```python
from build123d import *

# Parameters (mm, degrees)
BOSS_EXTRUDE1_DEPTH = 50
CUT_EXTRUDE1_REACH  = 64.546
SKETCH2_R           = 2.5
CUT_EXTRUDE2_REACH  = 63.384
SKETCH3_R           = 3
FILLET1_R           = 6


with BuildPart() as part:
    # Sketch1 → Boss-Extrude1 (new, symmetric)
    with BuildSketch(Plane.XY):
        Polygon((0, 34), (0, 0), (22, 0), (22, 6), (6, 6), (6, 34), align=None)
    extrude(amount=BOSS_EXTRUDE1_DEPTH, both=True)

    # Sketch2 → Cut-Extrude1 (cut, up to next)
    with BuildSketch(Plane(origin=(6, 0, 0), x_dir=(0, 0, -1), z_dir=(1, 0, 0)), mode=Mode.PRIVATE) as cut_extrude1_sk1:
        with Locations(Location((-37.5, 22, 0), (0, 0, 90))):
            Circle(SKETCH2_R)
    cut_extrude1_tool1 = extrude(cut_extrude1_sk1.sketch, amount=-CUT_EXTRUDE1_REACH, mode=Mode.PRIVATE) & part.part
    # Sketch2 → Cut-Extrude1 (cut, up to next)
    with BuildSketch(Plane(origin=(6, 0, 0), x_dir=(0, 0, -1), z_dir=(1, 0, 0)), mode=Mode.PRIVATE) as cut_extrude1_sk2:
        with Locations((37.5, 22)):
            Circle(SKETCH2_R)
    cut_extrude1_tool2 = extrude(cut_extrude1_sk2.sketch, amount=-CUT_EXTRUDE1_REACH, mode=Mode.PRIVATE) & part.part
    add(cut_extrude1_tool1.solids().sort_by_distance((6, 22, 37.5))[0], mode=Mode.SUBTRACT)
    add(cut_extrude1_tool2.solids().sort_by_distance((6, 22, -37.5))[0], mode=Mode.SUBTRACT)

    # Sketch3 → Cut-Extrude2 (cut, up to next)
    with BuildSketch(Plane(origin=(0, 6, 0), x_dir=(1, 0, 0), z_dir=(0, 1, 0)), mode=Mode.PRIVATE) as cut_extrude2_sk1:
        with Locations(Location((13.3, 0, 0), (0, 0, 180))):
            Circle(SKETCH3_R)
    cut_extrude2_tool1 = extrude(cut_extrude2_sk1.sketch, amount=-CUT_EXTRUDE2_REACH, mode=Mode.PRIVATE) & part.part
    add(cut_extrude2_tool1.solids().sort_by_distance((13.3, 6, 0))[0], mode=Mode.SUBTRACT)

    # Fillet1
    fillet1_edges = [part.edges().sort_by_distance(p)[0] for p in [
        (22, 3, 50),
        (3, 34, 50),
        (22, 3, -50),
        (3, 34, -50),
    ]]
    fillet(fillet1_edges, radius=FILLET1_R)


solid = part.part
```
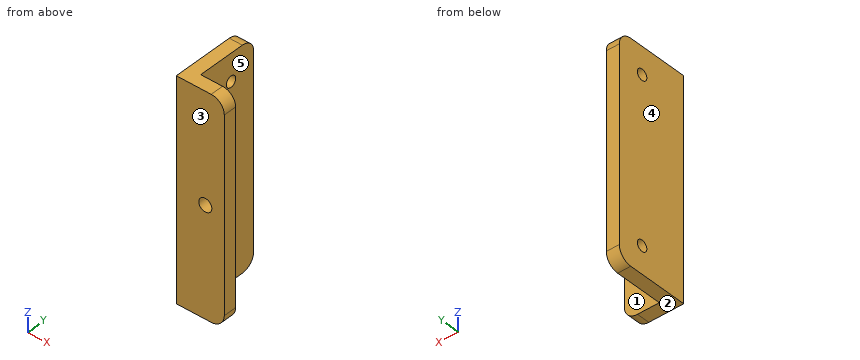
Input: part model. Units: mm. Frame: model coordinates. Face numbers are marked on the shaded views. A direction names the side the tool comes from. Round coordinates to 2 decimals unless told otherwise and drop trailing zeros. Loops run counter-clockwise (first coordinate to the right, second up) from the corner with the lowest first, then second, coordinate; pieces in that order, holes last.
1) Pull-direction query (Y, two-part tool) for the marked faces 1, 2 and 3; classes: released by +Y, released by -Y, zero draft, split by the parting line, or undercut.
Ans:
face 1: released by +Y
face 2: zero draft
face 3: released by -Y
2) Section query A-A on x = 13.3. Return the cut outline in (y, z).
Ans:
outline: (0, -50) - (6, -50) - (6, -3) - (0, -3) - close; (0, 3) - (6, 3) - (6, 50) - (0, 50) - close
3) Material intervals for line 1 (Y direction, x = 1.85, z = -37.5); line 2 (Z direction, x = 13.3, y = 4.4); line 3 (Y direction, x = 9.5, z = 19.5), sorted ascending.
Ans:
line 1: y = 0 to 19.5, 24.5 to 34
line 2: z = -50 to -3, 3 to 50
line 3: y = 0 to 6
4) Set-up query: the marked faces 4 and 5. Return all of +Z, -Z, +X, -X, +Y, -Y with unobstructed straight access to the full face (end or side cutting, diameter ignored); none if empty.
Ans:
face 4: +Z, -Z, -X, +Y, -Y
face 5: +Z, -Z, +X, +Y
5) Section query D-D on y = 3. Return the cut outline in (x, z).
Ans:
outline: (0, -50) - (16, -50) arc R6 ccw to (22, -44) - (22, 44) arc R6 ccw to (16, 50) - (0, 50) - close; hole circle Ø6 at (13.3, 0)
6) Section query C-C on y = 22. Return the cut outline in (x, z).
Ans:
outline: (0, -50) - (6, -50) - (6, -40) - (0, -40) - close; (0, -35) - (6, -35) - (6, 35) - (0, 35) - close; (0, 40) - (6, 40) - (6, 50) - (0, 50) - close
7) Pin query (flat end, axial travel): pin 1 (10 mm diameter, centred on y = 28.5, z = 10.5, fed in from -X); pin 2 (8.5 mm diameter, centred on y = 24.5, z = -23.5, fed in from +X); pin 3 (4.5 mm diameter, centred on y = 22, z = 37.5, fed in from +X); pin 4 (5 mm diameter, centred on x = 10.5, z = 6, fed in from +Y). Return the tip coordinate at first contact, or that it passes through.
Ans:
pin 1: stops at x = 0
pin 2: stops at x = 6
pin 3: passes through
pin 4: stops at y = 6
8) Section query B-B on z = 0. Return the cut outline in (x, y).
Ans:
outline: (0, 0) - (10.3, 0) - (10.3, 6) - (6, 6) - (6, 34) - (0, 34) - close; (16.3, 0) - (22, 0) - (22, 6) - (16.3, 6) - close
